Geometry check sheet. Reference: the model listing, model coordinates, mm. Round coordinates to 2 decimals unless told otherwise and drop trailing zeros. Write each loop counter-clockwise with the first axis right and the second up, starting at its lowest first coordinate (ties: lowest second). Pieces come first, ordered by that corner, then holes. Notation, with made-up numbers: (80.5, -33) - (134.5, -33) arc R17 ccw to (134.5, -3) - close; hole circle Ø10 at (-17, 67.25). An arc over 180 degrees is marked (long way). Return JSON: item names as keys, results as strings. Group by question number.
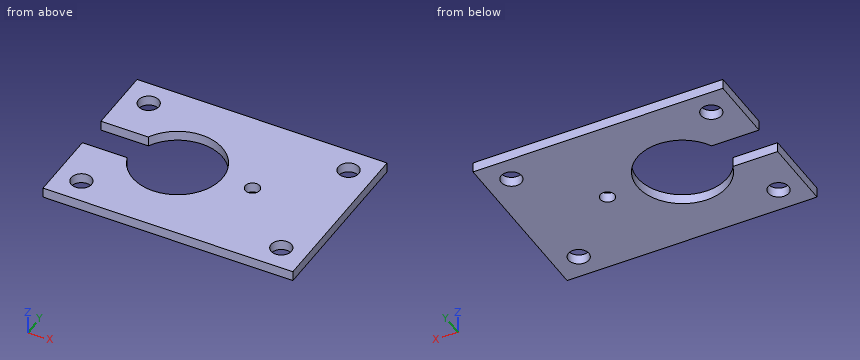
Autodesk Inventor part; units mm, degrees
ref_plane "YZ Plane" through (0, 0, 0) normal (1, 0, 0) x (0, 1, 0)
ref_plane "XZ Plane" through (0, 0, 0) normal (0, 1, 0) x (-1, 0, 0)
ref_plane "XY Plane" through (0, 0, 0) normal (0, 0, 1) x (1, 0, 0)
sketch "Skizze1" plane through (0, 0, 0) normal (0, 0, 1) x (1, 0, 0)
  line L0 (0, 0) -> (50, 0)
  line L1 (50, 0) -> (50, 35)
  line L2 (50, 35) -> (0, 35)
  line L3 (0, 35) -> (0, 0)
  circle A0 centre (17.5, 17.5) radius 1.05
  circle A1 centre (32.5, 17.5) radius 1.45
  line L4 (0, 17.5) -> (50, 17.5)
  line L5 (50, 0) -> (50, 17.5)
  line L6 (50, 17.5) -> (50, 35)
  line L7 (17.5, 17.5) -> (0, 17.5)
  line L8 (32.5, 17.5) -> (50, 17.5)
  dimension "d0" = 2.1
  dimension "d1" = 2.9
  dimension "d2" = 15
  dimension "d16" = 17.5
  dimension "d25" = 50
extrude "Extrusion1" add sketch "Skizze1" along normal blind 2 contours L3 L4 A0 A1 L1 L0 | L3 L2 L1 L4 A1 A0
sketch "Skizze5" plane through (0, 0, 2) normal (0, 0, 1) x (1, 0, 0)
  circle A0 centre (17.5, 17.5) radius 1.05
  circle A1 centre (17.5, 17.5) radius 9
  line L0 (10.0196, 14.6319) -> (-2.5086, 14.6319)
  line L1 (-2.5086, 14.6319) -> (-2.5086, 21.5511)
  line L2 (-2.5086, 21.5511) -> (10.0196, 21.5511)
  line L3 (10.0196, 21.5511) -> (10.0196, 14.6319)
  circle A2 centre (17.5, 17.5) radius 7.5
  dimension "d24" = 1.5
extrude "Extrusion5" cut sketch "Skizze5" against normal through all
sketch "Skizze6" plane through (0, 0, 2) normal (0, 0, 1) x (1, 0, 0)
  line L0 (0, 14.6319) -> (0, 0)
  line L1 (0, 0) -> (50, 0)
  line L2 (50, 0) -> (50, 35)
  line L3 (50, 35) -> (0, 35)
  line L4 (5, 30) -> (45, 30)
  line L5 (45, 30) -> (45, 5)
  line L6 (45, 5) -> (5, 5)
  line L7 (5, 5) -> (5, 30)
  dimension "d26" = 5
  dimension "d27" = 5
  dimension "d28" = 5
  dimension "d29" = 5
hole "Bohrung1" at (5, 5, 2) at (5, 30, 2) at (45, 30, 2) at (45, 5, 2) direction (0, 0, -1) diameter 4.1 end through all
properties part number "GehäuseFront"
1. Material ranges on line 1 along Y through (x, z) = (45, 1.25); line 2 along Y through (x, z) = (32.5, 0.5); line 3 along Y through (x, z) = (43.5, 0.5), recorded low to high.
2. Depth check by flat-ended pin: pin 1 Ø5.5 at (x, y) = (45, 5) entering from -Z; pin 2 Ø3 at (x, y) = (9, 20) entering from -Z. Enter the tip coordinate at first touch or a pass-through.
3. Section check C-C (y = 17.5). Enter the section's corners in (x, z).
4. Section check B-B (z = 1.3). Enter the section's corners in (x, y), and give its area (3 significant figures).
5. Section check D-D (y = 5). Enter the section's corners in (x, z), and give its area (3 significant figures).
6. Section check A-A (x = 32.5). Enter the section's corners in (y, z), and give its area (3 significant figures).
Result sheet:
{
 "1": {"line 1": "y = 0 to 2.95, 7.05 to 27.95, 32.05 to 35", "line 2": "y = 0 to 16.05, 18.95 to 35", "line 3": "y = 0 to 3.6, 6.4 to 28.6, 31.4 to 35"},
 "2": {"pin 1": "stops at z = 0", "pin 2": "passes through"},
 "3": {"outline": "(26.5, 0) - (31.05, 0) - (31.05, 2) - (26.5, 2) - close; (33.95, 0) - (50, 0) - (50, 2) - (33.95, 2) - close"},
 "4": {"outline": "(0, 0) - (50, 0) - (50, 35) - (0, 35) - (0, 21.55) - (9.46, 21.55) arc R9 cw (long way) to (8.97, 14.63) - (0, 14.63) - close; hole circle Ø4.1 at (5, 5); hole circle Ø4.1 at (5, 30); hole circle Ø2.9 at (32.5, 17.5); hole circle Ø4.1 at (45, 5); hole circle Ø4.1 at (45, 30)", "area": "1,380 mm²"},
 "5": {"outline": "(0, 0) - (2.95, 0) - (2.95, 2) - (0, 2) - close; (7.05, 0) - (42.95, 0) - (42.95, 2) - (7.05, 2) - close; (47.05, 0) - (50, 0) - (50, 2) - (47.05, 2) - close", "area": "83.6 mm²"},
 "6": {"outline": "(0, 0) - (16.05, 0) - (16.05, 2) - (0, 2) - close; (18.95, 0) - (35, 0) - (35, 2) - (18.95, 2) - close", "area": "64.2 mm²"}
}
